from build123d import *

# Parameters (mm, degrees)
SKETCH1_W               = 380
SKETCH1_H               = 200
BOSS_EXTRUDE1_DEPTH     = 6
SKETCH6_W               = 6
SKETCH6_H               = 20
CUT_EXTRUDE4_DEPTH      = 7
LPATTERN3_COUNT         = 5
LPATTERN3_PITCH         = 40
SKETCH7_W               = 20
SKETCH7_H               = 6
CUT_EXTRUDE5_DEPTH      = 10
LPATTERN4_COUNT         = 9
LPATTERN4_PITCH         = 40
MIRROR1_COPY_1_SKETCH_W = 20
MIRROR1_COPY_1_SKETCH_H = 6
MIRROR1_COPY_1_DEPTH    = 10
MIRROR1_COPY_2_SKETCH_W = 20
MIRROR1_COPY_2_SKETCH_H = 6
MIRROR1_COPY_2_DEPTH    = 10
MIRROR1_COPY_3_SKETCH_W = 20
MIRROR1_COPY_3_SKETCH_H = 6
MIRROR1_COPY_3_DEPTH    = 10
MIRROR1_COPY_4_SKETCH_W = 20
MIRROR1_COPY_4_SKETCH_H = 6
MIRROR1_COPY_4_DEPTH    = 10
MIRROR1_COPY_5_SKETCH_W = 20
MIRROR1_COPY_5_SKETCH_H = 6
MIRROR1_COPY_5_DEPTH    = 10
MIRROR1_COPY_6_SKETCH_W = 20
MIRROR1_COPY_6_SKETCH_H = 6
MIRROR1_COPY_6_DEPTH    = 10
MIRROR1_COPY_7_SKETCH_W = 20
MIRROR1_COPY_7_SKETCH_H = 6
MIRROR1_COPY_7_DEPTH    = 10
MIRROR1_COPY_8_SKETCH_W = 20
MIRROR1_COPY_8_SKETCH_H = 6
MIRROR1_COPY_8_DEPTH    = 10
MIRROR2_COPY_1_SKETCH_W = 6
MIRROR2_COPY_1_SKETCH_H = 20
MIRROR2_COPY_1_DEPTH    = 7
MIRROR2_COPY_2_SKETCH_W = 6
MIRROR2_COPY_2_SKETCH_H = 20
MIRROR2_COPY_2_DEPTH    = 7
MIRROR2_COPY_3_SKETCH_W = 6
MIRROR2_COPY_3_SKETCH_H = 20
MIRROR2_COPY_3_DEPTH    = 7
MIRROR2_COPY_4_SKETCH_W = 6
MIRROR2_COPY_4_SKETCH_H = 20
MIRROR2_COPY_4_DEPTH    = 7
SKETCH10_W              = 6
SKETCH10_H              = 20
CUT_EXTRUDE6_DEPTH      = 10
LPATTERN5_COUNT         = 5
LPATTERN5_PITCH         = 40
SKETCH11_W              = 20
SKETCH11_H              = 6
CUT_EXTRUDE7_DEPTH      = 10
LPATTERN6_COUNT         = 2
LPATTERN6_PITCH         = 40


with BuildPart() as part:
    # Sketch1 → Boss-Extrude1 (new body)
    with BuildSketch(Plane.XY):
        with Locations((77.096774194, -21.774193548)):
            Rectangle(SKETCH1_W, SKETCH1_H)
    extrude(amount=BOSS_EXTRUDE1_DEPTH)

    # Sketch6 → Cut-Extrude4 (cut, through all)
    with BuildSketch(Plane.XY):
        with Locations((-109.903225806, 68.225806452)):
            Rectangle(SKETCH6_W, SKETCH6_H)
    cut_extrude4 = extrude(amount=CUT_EXTRUDE4_DEPTH, mode=Mode.SUBTRACT)

    # LPattern3: Cut-Extrude4 ×5
    with Locations(*[(0, -i * LPATTERN3_PITCH, 0) for i in range(1, LPATTERN3_COUNT)]):
        add(cut_extrude4, mode=Mode.SUBTRACT)

    # Sketch7 → Cut-Extrude5 (cut)
    with BuildSketch(Plane.XY.offset(6)):
        with Locations((-82.903225806, 75.225806452)):
            Rectangle(SKETCH7_W, SKETCH7_H)
    cut_extrude5 = extrude(amount=-CUT_EXTRUDE5_DEPTH, mode=Mode.SUBTRACT)

    # LPattern4: Cut-Extrude5 ×9
    with Locations(*[(i * LPATTERN4_PITCH, 0, 0) for i in range(1, LPATTERN4_COUNT)]):
        add(cut_extrude5, mode=Mode.SUBTRACT)

    # Mirror1: Cut-Extrude5 across plane
    add(cut_extrude5.mirror(Plane.ZX.offset(-21.774193548)), mode=Mode.SUBTRACT)

    # Mirror1 copy 1 sketch → Mirror1 copy 1 (cut)
    with BuildSketch(Plane(origin=(40, -43.548387097, 6), x_dir=(1, 0, 0), z_dir=(0, 0, 1))):
        with Locations((-82.903225806, -75.225806452)):
            Rectangle(MIRROR1_COPY_1_SKETCH_W, MIRROR1_COPY_1_SKETCH_H)
    extrude(amount=-MIRROR1_COPY_1_DEPTH, mode=Mode.SUBTRACT)

    # Mirror1 copy 2 sketch → Mirror1 copy 2 (cut)
    with BuildSketch(Plane(origin=(80, -43.548387097, 6), x_dir=(1, 0, 0), z_dir=(0, 0, 1))):
        with Locations((-82.903225806, -75.225806452)):
            Rectangle(MIRROR1_COPY_2_SKETCH_W, MIRROR1_COPY_2_SKETCH_H)
    extrude(amount=-MIRROR1_COPY_2_DEPTH, mode=Mode.SUBTRACT)

    # Mirror1 copy 3 sketch → Mirror1 copy 3 (cut)
    with BuildSketch(Plane(origin=(120, -43.548387097, 6), x_dir=(1, 0, 0), z_dir=(0, 0, 1))):
        with Locations((-82.903225806, -75.225806452)):
            Rectangle(MIRROR1_COPY_3_SKETCH_W, MIRROR1_COPY_3_SKETCH_H)
    extrude(amount=-MIRROR1_COPY_3_DEPTH, mode=Mode.SUBTRACT)

    # Mirror1 copy 4 sketch → Mirror1 copy 4 (cut)
    with BuildSketch(Plane(origin=(160, -43.548387097, 6), x_dir=(1, 0, 0), z_dir=(0, 0, 1))):
        with Locations((-82.903225806, -75.225806452)):
            Rectangle(MIRROR1_COPY_4_SKETCH_W, MIRROR1_COPY_4_SKETCH_H)
    extrude(amount=-MIRROR1_COPY_4_DEPTH, mode=Mode.SUBTRACT)

    # Mirror1 copy 5 sketch → Mirror1 copy 5 (cut)
    with BuildSketch(Plane(origin=(200, -43.548387097, 6), x_dir=(1, 0, 0), z_dir=(0, 0, 1))):
        with Locations((-82.903225806, -75.225806452)):
            Rectangle(MIRROR1_COPY_5_SKETCH_W, MIRROR1_COPY_5_SKETCH_H)
    extrude(amount=-MIRROR1_COPY_5_DEPTH, mode=Mode.SUBTRACT)

    # Mirror1 copy 6 sketch → Mirror1 copy 6 (cut)
    with BuildSketch(Plane(origin=(240, -43.548387097, 6), x_dir=(1, 0, 0), z_dir=(0, 0, 1))):
        with Locations((-82.903225806, -75.225806452)):
            Rectangle(MIRROR1_COPY_6_SKETCH_W, MIRROR1_COPY_6_SKETCH_H)
    extrude(amount=-MIRROR1_COPY_6_DEPTH, mode=Mode.SUBTRACT)

    # Mirror1 copy 7 sketch → Mirror1 copy 7 (cut)
    with BuildSketch(Plane(origin=(280, -43.548387097, 6), x_dir=(1, 0, 0), z_dir=(0, 0, 1))):
        with Locations((-82.903225806, -75.225806452)):
            Rectangle(MIRROR1_COPY_7_SKETCH_W, MIRROR1_COPY_7_SKETCH_H)
    extrude(amount=-MIRROR1_COPY_7_DEPTH, mode=Mode.SUBTRACT)

    # Mirror1 copy 8 sketch → Mirror1 copy 8 (cut)
    with BuildSketch(Plane(origin=(320, -43.548387097, 6), x_dir=(1, 0, 0), z_dir=(0, 0, 1))):
        with Locations((-82.903225806, -75.225806452)):
            Rectangle(MIRROR1_COPY_8_SKETCH_W, MIRROR1_COPY_8_SKETCH_H)
    extrude(amount=-MIRROR1_COPY_8_DEPTH, mode=Mode.SUBTRACT)

    # Mirror2: Cut-Extrude4 across plane
    add(cut_extrude4.mirror(Plane(origin=(77.096774194, 0, 0), x_dir=(0, 0, 1), z_dir=(1, 0, 0))), mode=Mode.SUBTRACT)

    # Mirror2 copy 1 sketch → Mirror2 copy 1 (cut, through all)
    with BuildSketch(Plane(origin=(154.193548387, -40, 0), x_dir=(-1, 0, 0), z_dir=(0, 0, 1))):
        with Locations((-109.903225806, -68.225806452)):
            Rectangle(MIRROR2_COPY_1_SKETCH_W, MIRROR2_COPY_1_SKETCH_H)
    extrude(amount=MIRROR2_COPY_1_DEPTH, mode=Mode.SUBTRACT)

    # Mirror2 copy 2 sketch → Mirror2 copy 2 (cut, through all)
    with BuildSketch(Plane(origin=(154.193548387, -80, 0), x_dir=(-1, 0, 0), z_dir=(0, 0, 1))):
        with Locations((-109.903225806, -68.225806452)):
            Rectangle(MIRROR2_COPY_2_SKETCH_W, MIRROR2_COPY_2_SKETCH_H)
    extrude(amount=MIRROR2_COPY_2_DEPTH, mode=Mode.SUBTRACT)

    # Mirror2 copy 3 sketch → Mirror2 copy 3 (cut, through all)
    with BuildSketch(Plane(origin=(154.193548387, -120, 0), x_dir=(-1, 0, 0), z_dir=(0, 0, 1))):
        with Locations((-109.903225806, -68.225806452)):
            Rectangle(MIRROR2_COPY_3_SKETCH_W, MIRROR2_COPY_3_SKETCH_H)
    extrude(amount=MIRROR2_COPY_3_DEPTH, mode=Mode.SUBTRACT)

    # Mirror2 copy 4 sketch → Mirror2 copy 4 (cut, through all)
    with BuildSketch(Plane(origin=(154.193548387, -160, 0), x_dir=(-1, 0, 0), z_dir=(0, 0, 1))):
        with Locations((-109.903225806, -68.225806452)):
            Rectangle(MIRROR2_COPY_4_SKETCH_W, MIRROR2_COPY_4_SKETCH_H)
    extrude(amount=MIRROR2_COPY_4_DEPTH, mode=Mode.SUBTRACT)

    # Sketch10 → Cut-Extrude6 (cut)
    with BuildSketch(Plane(origin=(0, 0, 0), x_dir=(-1, 0, 0), z_dir=(0, 0, -1))):
        with Locations((15.903225806, 68.225806452)):
            Rectangle(SKETCH10_W, SKETCH10_H)
    cut_extrude6 = extrude(amount=-CUT_EXTRUDE6_DEPTH, mode=Mode.SUBTRACT)

    # LPattern5: Cut-Extrude6 ×5
    with Locations(*[(0, -i * LPATTERN5_PITCH, 0) for i in range(1, LPATTERN5_COUNT)]):
        add(cut_extrude6, mode=Mode.SUBTRACT)

    # Sketch11 → Cut-Extrude7 (cut)
    with BuildSketch(Plane(origin=(0, 0, 0), x_dir=(-1, 0, 0), z_dir=(0, 0, -1))):
        with Locations((42.903225806, -38.774193548)):
            Rectangle(SKETCH11_W, SKETCH11_H)
    cut_extrude7 = extrude(amount=-CUT_EXTRUDE7_DEPTH, mode=Mode.SUBTRACT)

    # LPattern6: Cut-Extrude7 ×2
    with Locations(*[(-i * LPATTERN6_PITCH, 0, 0) for i in range(1, LPATTERN6_COUNT)]):
        add(cut_extrude7, mode=Mode.SUBTRACT)


solid = part.part
Geometry: final body of the model. Coordinates: model frame, mm. Give positions to 0.01 mm unless a question says otherwise; leave off trailing zeros. Write each loop counter-clockwise with the first axis right and the second up, starting at its lowest first coordinate (ties: lowest second). Pieces come first, ordered by that corner, then holes. Notation, with made-up numbers: M 60,25.25 L 97,25.25 A23 ccw 97,46.25 Z; hole C -37.75,86.5 d11. An arc over 180 degrees is marked long. Answer in a Markdown table with one row per item. Add a question column.
(1) Ray query, line 1 (X direction, y = -39, z = 4.7); line 2 (Y direction, x = -16.5, z = 1.8); line 3 (X direction, y = -43, z = 3.9). Return the intervals inside material, ascending.
(2) Section C-C on z = 0.9. State how many separate pieces and enclosed holes the cut face has, and give its area (3 significant figures).
(3) First-contact query: pin 1 (1.8 mm diameter, centred on y = 76, z = 4, fed in from +X); pin 2 (1.8 mm diameter, centred on x = -43, z = 2.5, fed in from +Y); pin 3 (1 mm diameter, centred on y = -100.5, z = 3, fed in from -X). Flat tips, straight axial feed; report the tip coordinate or a pass-through.
(4) Section A-A on y = -16.5. Return loops of the section in (x, z).
(5) Section B-B on x = -85.5. Return loops of the section in (y, z).
(6) Section D-D on x = 74. Return loops of the section in (y, z).
Result set:
| question | item | result |
|---|---|---|
| 1 | line 1 | x = -112.9 to -92.9, -72.9 to -52.9, -32.9 to 267.1 |
| 1 | line 2 | y = -121.77 to -101.77, -81.77 to -61.77, -41.77 to -21.77, -1.77 to 18.23, 38.23 to 58.23 |
| 1 | line 3 | x = -106.9 to -18.9, -12.9 to 261.1 |
| 2 | separate pieces | 1 |
| 2 | enclosed holes | 6 |
| 2 | area | 71,800 mm^2 |
| 3 | pin 1 | stops at x = 261.1 |
| 3 | pin 2 | stops at y = 72.23 |
| 3 | pin 3 | stops at x = -106.9 |
| 4 | outline | M -106.9,0 L -18.9,0 L -18.9,6 L -106.9,6 Z; M -12.9,0 L 261.1,0 L 261.1,6 L -12.9,6 Z |
| 5 | outline | M -115.77,0 L -41.77,0 L -41.77,6 L -115.77,6 Z; M -35.77,0 L 72.23,0 L 72.23,6 L -35.77,6 Z |
| 6 | outline | M -115.77,0 L 72.23,0 L 72.23,6 L -115.77,6 Z |
